```python
from build123d import *

# Parameters (mm, degrees)
SKETCH1_W               = 4.2
SKETCH1_H               = 17.5
BOSS_EXTRUDE1_DEPTH     = 1.2
SKETCH2_W               = 1
SKETCH2_H               = 17.5
BOSS_EXTRUDE2_DEPTH     = 5
CUT_EXTRUDE1_DEPTH      = 1.3
CUT_EXTRUDE1_DEPTH_BACK = 5
SKETCH4_W               = 4
SKETCH4_H               = 3
BOSS_EXTRUDE3_DEPTH     = 1
SKETCH5_R               = 0.5125
CUT_EXTRUDE2_DEPTH      = 2.2
SKETCH6_R               = 0.5
CUT_EXTRUDE3_DEPTH      = 0.75
SKETCH11_R              = 0.15
CUT_EXTRUDE5_DEPTH      = 1.3
CUT_EXTRUDE5_DEPTH_BACK = 5.2
CUT_EXTRUDE7_DEPTH      = 0.2
CUT_EXTRUDE6_DEPTH      = 1.3
CUT_EXTRUDE6_DEPTH_BACK = 1.3
SKETCH14_W              = 1.5
SKETCH14_H              = 4.2
SKETCH14_H_2            = 6.2
SKETCH14_W_2            = 0.5
SKETCH14_H_3            = 9.2
BOSS_EXTRUDE5_DEPTH     = 0.2
FILLET1_R               = 0.5
CUT_EXTRUDE8_DEPTH      = 0.6


with BuildPart() as part:
    # Sketch1 → Boss-Extrude1 (new body)
    with BuildSketch(Plane(origin=(0, 0, 0), x_dir=(1, 0, 0), z_dir=(0, 1, 0))):
        with Locations((2.1, 8.75)):
            Rectangle(SKETCH1_W, SKETCH1_H)
    extrude(amount=BOSS_EXTRUDE1_DEPTH)

    # Sketch2 → Boss-Extrude2 (add)
    with BuildSketch(Plane(origin=(0, 1.2, 0), x_dir=(1, 0, 0), z_dir=(0, 1, 0))):
        with Locations((3.7, 8.75)):
            Rectangle(SKETCH2_W, SKETCH2_H)
    extrude(amount=BOSS_EXTRUDE2_DEPTH)

    # Sketch3 → Cut-Extrude1 (cut, two sides)
    with BuildSketch(Plane(origin=(4.2, 0, 0), x_dir=(0, 0, -1), z_dir=(1, 0, 0))) as cut_extrude1_sk:
        Polygon((0, 4.2), (0, 6.2), (2.236067977, 6.2), align=None)
        Polygon((17.5, 6.2), (15.263932023, 6.2), (17.5, 4.2), align=None)
    extrude(amount=CUT_EXTRUDE1_DEPTH, mode=Mode.SUBTRACT)
    extrude(cut_extrude1_sk.sketch, amount=-CUT_EXTRUDE1_DEPTH_BACK, mode=Mode.SUBTRACT)

    # Sketch4 → Boss-Extrude3 (add)
    with BuildSketch(Plane(origin=(4.2, 0, 0), x_dir=(0, 0, -1), z_dir=(1, 0, 0))):
        with Locations((8.236067977, 7.7)):
            Rectangle(SKETCH4_W, SKETCH4_H)
    extrude(amount=-BOSS_EXTRUDE3_DEPTH)

    # Sketch5 → Cut-Extrude2 (cut, through all)
    with BuildSketch(Plane(origin=(0, 1.2, 0), x_dir=(1, 0, 0), z_dir=(0, 1, 0))):
        with Locations((1.2, 16.3)):
            Circle(SKETCH5_R)
        with Locations((1.2, 1.2)):
            Circle(SKETCH5_R)
    extrude(amount=-CUT_EXTRUDE2_DEPTH, mode=Mode.SUBTRACT)

    # Sketch6 → Cut-Extrude3 (cut)
    with BuildSketch(Plane(origin=(0, 1.2, 0), x_dir=(1, 0, 0), z_dir=(0, 1, 0))):
        with Locations((1.4, 8.8)):
            Circle(SKETCH6_R)
    extrude(amount=-CUT_EXTRUDE3_DEPTH, mode=Mode.SUBTRACT)

    # Sketch11 → Cut-Extrude5 (cut, two sides)
    with BuildSketch(Plane(origin=(4.2, 0, 0), x_dir=(0, 0, -1), z_dir=(1, 0, 0))) as cut_extrude5_sk:
        with Locations((3.5, 5.40229833)):
            Circle(SKETCH11_R)
        with Locations((6.191844332, 5.3)):
            Circle(SKETCH11_R)
        with Locations((3.5, 2)):
            Circle(SKETCH11_R)
        with Locations((11.308155668, 5.3)):
            Circle(SKETCH11_R)
        with Locations((14, 5.4)):
            Circle(SKETCH11_R)
        with Locations((14, 2)):
            Circle(SKETCH11_R)
    extrude(amount=CUT_EXTRUDE5_DEPTH, mode=Mode.SUBTRACT)
    extrude(cut_extrude5_sk.sketch, amount=-CUT_EXTRUDE5_DEPTH_BACK, mode=Mode.SUBTRACT)

    # Sketch15 → Cut-Extrude7 (cut)
    with BuildSketch(Plane.ZY.offset(-3.2)):
        Polygon((-14, 5.75), (-14.303108891, 5.575), (-14.303108891, 5.225), (-14, 5.05), (-13.696891109, 5.225), (-13.696891109, 5.575), align=None)
        Polygon((-11.308155668, 5.65), (-11.611264559, 5.475), (-11.611264559, 5.125), (-11.308155668, 4.95), (-11.005046777, 5.125), (-11.005046777, 5.475), align=None)
        Polygon((-14, 2.35), (-14.303108891, 2.175), (-14.303108891, 1.825), (-14, 1.65), (-13.696891109, 1.825), (-13.696891109, 2.175), align=None)
        Polygon((-6.191844332, 5.65), (-6.494953223, 5.475), (-6.494953223, 5.125), (-6.191844332, 4.95), (-5.888735441, 5.125), (-5.888735441, 5.475), align=None)
        Polygon((-3.5, 5.75229833), (-3.803108891, 5.57729833), (-3.803108891, 5.22729833), (-3.5, 5.05229833), (-3.196891109, 5.22729833), (-3.196891109, 5.57729833), align=None)
        Polygon((-3.5, 2.35), (-3.803108891, 2.175), (-3.803108891, 1.825), (-3.5, 1.65), (-3.196891109, 1.825), (-3.196891109, 2.175), align=None)
    extrude(amount=-CUT_EXTRUDE7_DEPTH, mode=Mode.SUBTRACT)

    # Sketch12 → Cut-Extrude6 (cut, two sides)
    with BuildSketch(Plane(origin=(4.2, 0, 0), x_dir=(0, 0, -1), z_dir=(1, 0, 0))) as cut_extrude6_sk:
        with BuildLine():
            Line((8.886067977, 8.2), (8.886067977, 1.5))
            ThreePointArc((8.886067977, 1.5), (8.736067977, 1.35), (8.586067977, 1.5))
            Line((8.586067977, 1.5), (8.586067977, 8.2))
            ThreePointArc((8.586067977, 8.2), (8.736067977, 8.35), (8.886067977, 8.2))
        make_face()
        with BuildLine():
            Line((7.086067977, 8.2), (7.086067977, 1.5))
            ThreePointArc((7.086067977, 1.5), (6.936067977, 1.35), (6.786067977, 1.5))
            Line((6.786067977, 1.5), (6.786067977, 8.2))
            ThreePointArc((6.786067977, 8.2), (6.936067977, 8.35), (7.086067977, 8.2))
        make_face()
    extrude(amount=CUT_EXTRUDE6_DEPTH, mode=Mode.SUBTRACT)
    extrude(cut_extrude6_sk.sketch, amount=-CUT_EXTRUDE6_DEPTH_BACK, mode=Mode.SUBTRACT)

    # Sketch14 → Boss-Extrude5 (add)
    with BuildSketch(Plane(origin=(4.2, 0, 0), x_dir=(0, 0, -1), z_dir=(1, 0, 0))):
        with Locations((0.75, 2.1)):
            Rectangle(SKETCH14_W, SKETCH14_H)
        Polygon((1.5, 4.2), (1.5, 5.541640786), (0, 4.2), align=None)
        with Locations((4.75, 3.1)):
            Rectangle(SKETCH14_W, SKETCH14_H_2)
        with Locations((12.75, 3.1)):
            Rectangle(SKETCH14_W, SKETCH14_H_2)
        with Locations((7.986067977, 4.6)):
            Rectangle(SKETCH14_W_2, SKETCH14_H_3)
        with Locations((16.75, 2.1)):
            Rectangle(SKETCH14_W, SKETCH14_H)
    extrude(amount=BOSS_EXTRUDE5_DEPTH)

    # Fillet1
    fillet1_edges = [part.edges().sort_by_distance(p)[0] for p in [
        (0, 1.2, -8.75),
    ]]
    fillet(fillet1_edges, radius=FILLET1_R)

    # Sketch16 → Cut-Extrude8 (cut)
    with BuildSketch(Plane(origin=(4.2, 0, 0), x_dir=(0, 0, -1), z_dir=(1, 0, 0))):
        with BuildLine():
            Line((8.336067977, 1.5), (8.336067977, 8.2))
            ThreePointArc((8.336067977, 8.2), (8.736067977, 8.6), (9.136067977, 8.2))
            Line((9.136067977, 8.2), (9.136067977, 1.5))
            ThreePointArc((9.136067977, 1.5), (8.736067977, 1.1), (8.336067977, 1.5))
        make_face()
        with BuildLine():
            Line((6.536067977, 1.5), (6.536067977, 8.2))
            ThreePointArc((6.536067977, 8.2), (6.936067977, 8.6), (7.336067977, 8.2))
            Line((7.336067977, 8.2), (7.336067977, 1.5))
            ThreePointArc((7.336067977, 1.5), (6.936067977, 1.1), (6.536067977, 1.5))
        make_face()
    extrude(amount=-CUT_EXTRUDE8_DEPTH, mode=Mode.SUBTRACT)


solid = part.part
```
Could you check a few things on this model? Use its own coordinates, in mm. A direction names the side the tool comes from. Coordinates: 2 decimals unless noted, no trailing zeros. Write each loop counter-clockwise with the first axis right and the second up, starting at its lowest first coordinate (ties: lowest second). Pieces come first, ordered by that corner, then holes. Notation, with made-up numbers: M 21,67 L 34,67 A32 cw 34,102 Z; hole C 6,19.5 d8. An arc over 180 degrees is marked long. Answer as CSV lines item,"result". Start each with the question number.
1) We'd pull the mould along Z, two halves only. Please class faces 1 (the flat face through (2, 0, -9)), 2 (the flat face through (1.4, 0.45, -8.8)), 3 (the flat face through (3.71, 5.21, -16.37)): +Z half, -Z half, draft (parallel to the pull), parting line (faces both ways), or undercut.
2) I want a section at D-D, the plane x = 3.9. Give the number of separate pieces and of enclosed holes in the cut face, and give its area (3 significant figures).
3) I want a section at C-C, the plane x = 1.4. Please give me the cut outline in (y, z).
4) For P1, Ø0.5, axis at y = 5.5, z = -14, coming from the -X side; P2, Ø1.6, axis at x = 1.2, z = -1.2, coming from the +Y side; P3, Ø0.7, axis at x = 4, y = 5, coming from the +Z side, each with a flat end and sliding along its axis, tell me the tip position at first contact or that it passes through.
5) I want a section at A-A, the plane y = 7. Please give me the cut outline in (x, z).
6) Please list where these lines run through material, in increasing order: line 1 (Y direction, x = 4, z = -3.5); line 2 (Z direction, x = 1.2, y = 0.4); line 3 (Z direction, x = 1.4, y = 0.7). Write a range as from..to.
7) I want a section at B-B, the plane z = -2.75. Please give me the cut outline in (x, y).
8) For faces 4 (the flat face through (3.2, 4, -11)), 5 (the flat face through (4, 8, -6.236)), 6 (the flat face through (4.2, 3, -3)), 7 (the cylindrical face through (1.631, 0.83, -8.356)), which set-ups out of +Z, -Z, +X, -X, +Y, -Y let a thin tool reach every point of the face, with its end or its side?
Data:
1,face 1,"draft"
1,face 2,"undercut"
1,face 3,"-Z half"
2,separate pieces,"1"
2,enclosed holes,"8"
2,area,"104 mm^2"
3,outline,"M 0,-17.5 L 1.2,-17.5 L 1.2,-16.77 L 0,-16.77 Z; M 0,-15.83 L 1.2,-15.83 L 1.2,-9.3 L 0.45,-9.3 L 0.45,-8.3 L 1.2,-8.3 L 1.2,-1.67 L 0,-1.67 Z; M 0,-0.73 L 1.2,-0.73 L 1.2,0 L 0,0 Z"
4,P1,"stops at x = 3.2"
4,P2,"stops at y = 1.2"
4,P3,"stops at z = -0.5"
5,outline,"M 3.2,-10.24 L 4.2,-10.24 L 4.2,-9.14 L 3.6,-9.14 L 3.6,-8.89 L 3.2,-8.89 Z; M 3.2,-8.59 L 3.6,-8.59 L 3.6,-8.34 L 4.2,-8.34 L 4.2,-8.24 L 4.4,-8.24 L 4.4,-7.74 L 4.2,-7.74 L 4.2,-7.34 L 3.6,-7.34 L 3.6,-7.09 L 3.2,-7.09 Z; M 3.2,-6.79 L 3.6,-6.79 L 3.6,-6.54 L 4.2,-6.54 L 4.2,-6.24 L 3.2,-6.24 Z"
6,line 1,"y = 0..1.85, 2.15..5.25, 5.55..6.2"
6,line 2,"z = -17.5..-16.81, -15.79..-1.71, -0.69..0"
6,line 3,"z = -17.5..-16.77, -15.83..-9.3, -8.3..-1.67, -0.73..0"
7,outline,"M 0,0 L 4.2,0 L 4.2,6.2 L 3.2,6.2 L 3.2,1.2 L 0.5,1.2 A0.5 ccw 0,0.7 Z"
8,face 4,"+Z, -Z, -X, +Y"
8,face 5,"+Z, +X, -X, +Y"
8,face 6,"+X, +Y, -Y"
8,face 7,"+Y"
